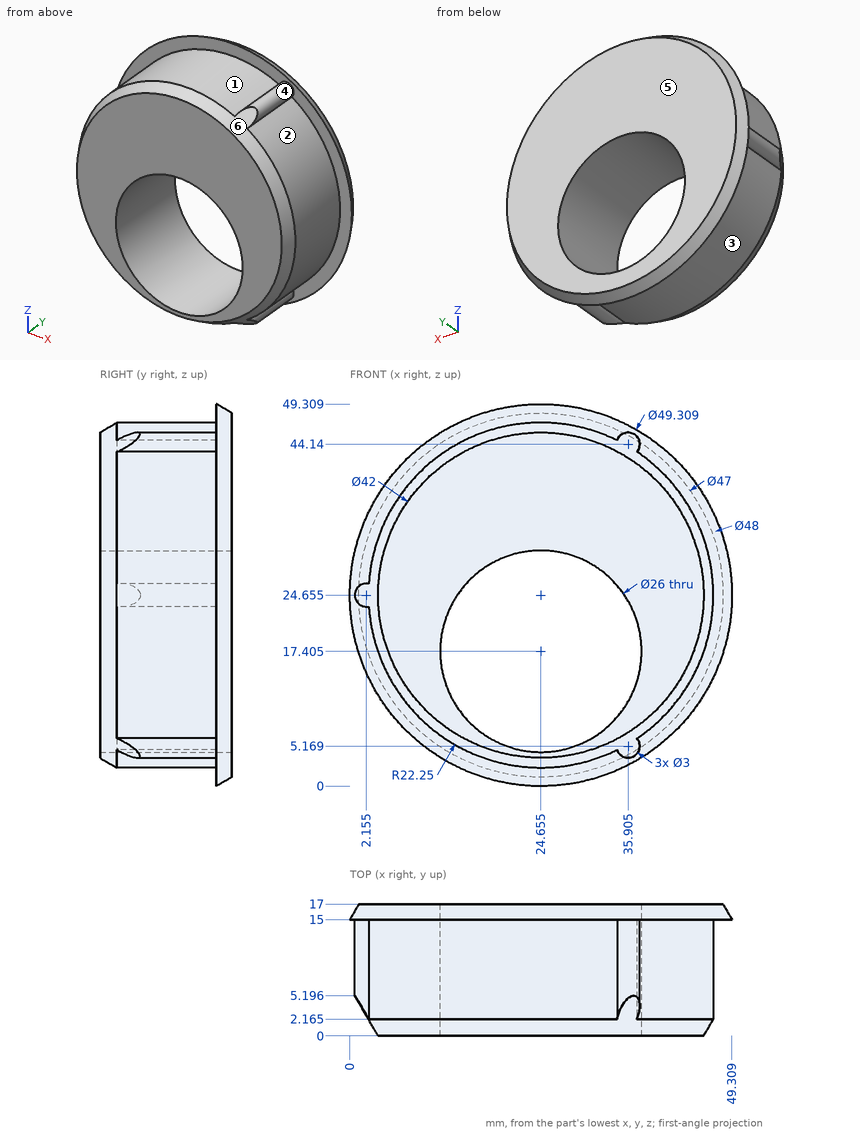
Here's the drawing with two shaded views (mm, measured from the low corner). I have some questions. A direction names the side the tool comes from. Give positions to 0.01 mm unless a question says otherwise; leave off trailing zeros. One line per item, written item: value. Start each with the question number.
1. For the marked faces 1, 2 and 3, which set-ups out of +Z, -Z, +X, -X, +Y, -Y let a thin tool reach every point of the face, with its end or its side?
2. I need wall thicknesses on probe 1 along X at (y, z) = (13.5, 12) (1 decimal); probe 2 along X at (y, z) = (4, 15); probe 3 along Z at (x, y) = (18, 15.5) (1 decimal). Which ranges of each line are inside material? Lowest first, please. Write a range as from..to.
3. Will these pins go through, and if not, where does the flat tip stop? pin 1 Ø2 at (x, y) = (44.5, 5.5) entering from +Z (1 decimal); pin 2 Ø2 at (y, z) = (6.5, 37.5) entering from -X; pin 3 Ø1 at (x, y) = (25.5, 9.5) entering from +Z.
4. We'd pull the mould along X, two halves only. Please class the marked faces 4, 5 and 6: released by +X, released by -X, zero draft, split by the parting line, or undercut.
Values follow:
1. face 1: +Z, -Y
1. face 2: +X, -Y
1. face 3: -Z, -Y
2. probe 1: x = 6.4..12.8, 36.5..43
2. probe 2: x = 4.61..11.88, 37.43..44.7
2. probe 3: z = 1.2..6.2, 28.6..48.1
3. pin 1: stops at z = 36.5
3. pin 2: stops at x = 5.82
3. pin 3: stops at z = 46.9
4. face 4: undercut
4. face 5: zero draft
4. face 6: split by the parting line
